```python
from build123d import *

# Parameters (mm, degrees)
F0_W           = 46.5
F0_H           = 42
F0_W_2         = 36.5
F0_H_2         = 36.5
F1_DEPTH       = 6.85
F2_DEPTH       = 1.66
F4_D           = 0.1
F4_CSINK_D     = 0.5
F4_CSINK_ANGLE = 90


with BuildPart() as f1:
    # F0 (on Front) → F1 (new body)
    with BuildSketch(Plane.XZ):
        with Locations((-23.25, 21)):
            Rectangle(F0_W, F0_H)
        with Locations((-23.25, 21)):
            Rectangle(F0_W_2, F0_H_2, mode=Mode.SUBTRACT)
        with Locations((-23.25, 21)):
            Rectangle(F0_W_2, F0_H_2)
    extrude(amount=F1_DEPTH)

    # F0 (on Front) → F2 (cut)
    with BuildSketch(Plane.XZ):
        with Locations((-23.25, 21)):
            Rectangle(F0_W_2, F0_H_2)
    extrude(amount=F2_DEPTH, mode=Mode.SUBTRACT)

    # F4 (through all)
    with Locations(Plane(origin=(0, -1.66, 0), x_dir=(-1, 0, 0), z_dir=(0, 1, 0))):
        with Locations((23.25, 21)):
            CounterSinkHole(F4_D / 2, F4_CSINK_D / 2, counter_sink_angle=F4_CSINK_ANGLE)


solid = f1.part
```
Geometry: final body of the model. Coordinates: model frame, mm. A direction names the side the tool comes from. Give positions to 0.01 mm unless a question says otherwise; leave off trailing zeros. Order: outer loops, then holes, each group sorted by start corner. A loop starts at its lowest first (then second) coordinate and runs counter-clockwise, first axis right, second up. Notation, with made-up numbers: (-21, 49.5) -> (-4, 49.5) arc R29 ccw to (-4, 69.5) -> close; hole circle Ø9 at (69, 88). An arc over 180 degrees is marked (long way). Write each question's results on one line, items separated by ' | '. Start each with the question number.
1) Draft query along Z for faces 3 (the flat face through (-24, -3, 0)), 4 (the flat face through (-24, -1.66, 21)), 5 (the flat face through (-24, -6.85, 21)). Return one class per face: pulls with the +Z half, pulls with the -Z half, needs draft (parallel to the pull), parting line crosses it, or undercut.
2) Line query: line 1 (X direction, y = -1, z = 6.5); line 2 (Z direction, x = -25.5, y = -1); line 3 (Y direction, x = -11, z = 23). Output: solid intervals per line, ascending. Write a range as from..to.
3) Set-up query: faces 1 (the flat face through (-24, 0, 40)), 2 (the flat face through (-24, -1, 39.25)). Return all of +Z, -Z, +X, -X, +Y, -Y with unobstructed straight access to the full face (end or side cutting, diameter ignored); none if empty.
4) Section B-B (z = 3.5). Return loops of the section in (x, y).
5) Section A-A (x = -7). Return loops of the section in (y, z).
Calculated:
1) face 3: pulls with the -Z half | face 4: undercut | face 5: needs draft
2) line 1: -46.5..-41.5, -5..0 | line 2: 0..2.75, 39.25..42 | line 3: -6.85..-1.66
3) face 1: +Z, -Z, +X, -X, +Y | face 2: +Y
4) outline: (-46.5, -6.85) -> (0, -6.85) -> (0, 0) -> (-5, 0) -> (-5, -1.66) -> (-41.5, -1.66) -> (-41.5, 0) -> (-46.5, 0) -> close
5) outline: (-6.85, 0) -> (0, 0) -> (0, 2.75) -> (-1.66, 2.75) -> (-1.66, 39.25) -> (0, 39.25) -> (0, 42) -> (-6.85, 42) -> close
